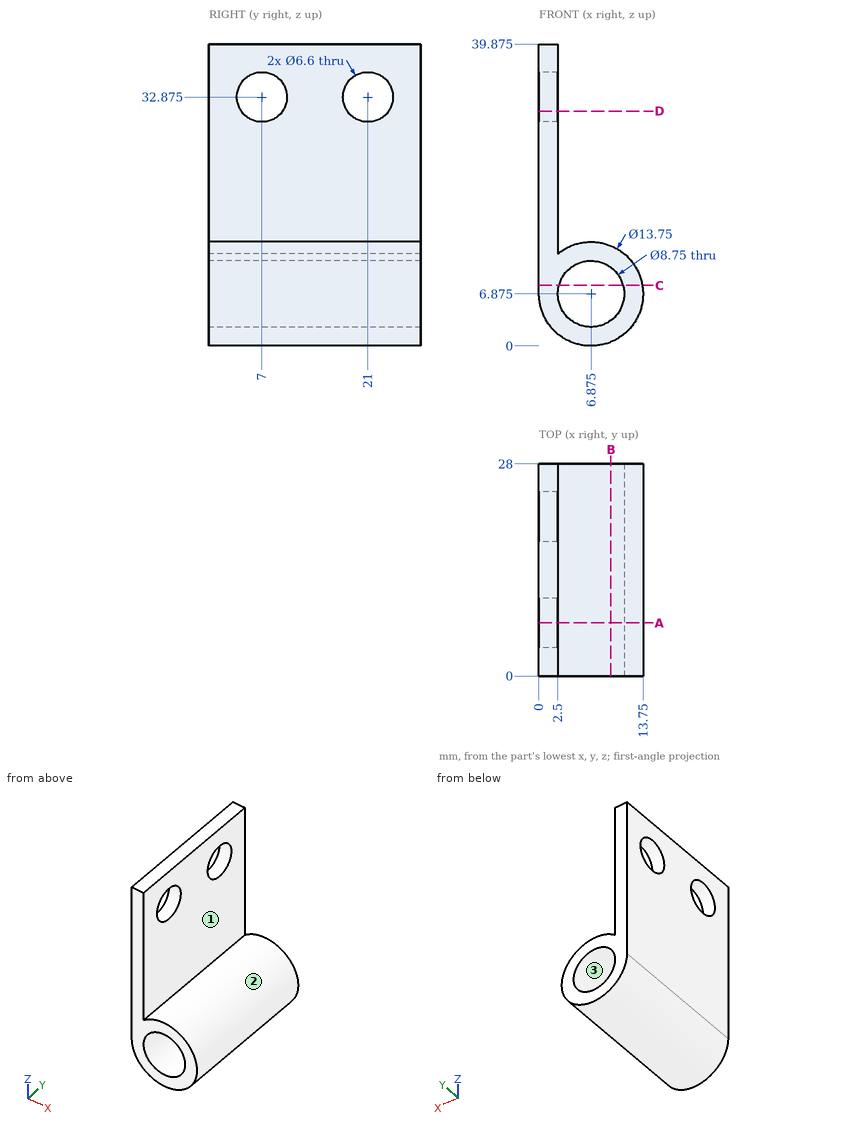
Geometry: see drawing. Coordinates: mm, zero at the bounding-box minimum. Give positions to 0.01 mm unless a question says otherwise; leave off trailing zeros. Write each loop counter-clockwise with the first axis right and the second up, starting at its lowest first coordinate (ties: lowest second). Pieces come first, ordered by that corner, then holes. Notation, with made-up numbers: M 35,33.25 L 57,33.25 A37 cw 57,72.25 Z; hole C -33,0 d5. An arc over 180 degrees is marked long. Answer in a Markdown table with one row per item. Add a question column.
(1) Mould query, pull axis Z, two halves, no side actions, for the marked faces 1, 2 and 3. Classes: +Z half, -Z half, draft (parallel to the pull), parting line (faces both ways), or undercut.
(2) Ray query, line 1 (X direction, y = 16, z = 34.5); line 2 (Z direction, x = 7, y = 23.5); line 3 (Z direction, x = 4, y = 19.5). Return the intervals inside material, ascending.
(3) Section B-B on x = 9.5. Return loops of the section in (y, z) (3 decimals).
(4) Section C-C on z = 8. Return loops of the section in (x, y), and give its area (3 significant figures).
(5) Section D-D on z = 31. Return loops of the section in (x, y), and give its area (3 significant figures).
(6) Section A-A on y = 7. Return loops of the section in (x, z) (3 decimals).
(7) First-contact query: pin 1 (7.5 mm diameter, centred on y = 21, z = 32.875, fed in from +X); pin 2 (1.5 mm diameter, centred on x = 10.5, y = 12, fed in from +Z); pin 3 (6 mm diameter, centred on y = 7, z = 32.875, fed in from +X) (3 decimals); pin 4 (1 mm diameter, centred on x = 5.5, y = 14, fed in from +Z). Flat tips, straight axial feed; report the tip coordinate or a pass-through.
Result set:
| question | item | result |
|---|---|---|
| 1 | face 1 | draft |
| 1 | face 2 | parting line |
| 1 | face 3 | undercut |
| 2 | line 1 | x = 0 to 2.5 |
| 2 | line 2 | z = 0 to 2.5, 11.25 to 13.75 |
| 2 | line 3 | z = 0.63 to 3.58, 10.17 to 13.12 |
| 3 | outline | M 0,0.521 L 28,0.521 L 28,3.375 L 0,3.375 Z; M 0,10.375 L 28,10.375 L 28,13.229 L 0,13.229 Z |
| 4 | outline | M 0,0 L 2.65,0 L 2.65,28 L 0,28 Z; M 11.1,0 L 13.66,0 L 13.66,28 L 11.1,28 Z |
| 4 | area | 146 mm^2 |
| 5 | outline | M 0,0 L 2.5,0 L 2.5,4.28 L 0,4.28 Z; M 0,9.72 L 2.5,9.72 L 2.5,18.28 L 0,18.28 Z; M 0,23.72 L 2.5,23.72 L 2.5,28 L 0,28 Z |
| 5 | area | 42.8 mm^2 |
| 6 | outline | M 0,6.875 A6.875 ccw long 2.5,12.178 L 2.5,29.575 L 0,29.575 Z; M 0,36.175 L 2.5,36.175 L 2.5,39.875 L 0,39.875 Z; hole C 6.875,6.875 d8.75 |
| 7 | pin 1 | stops at x = 2.5 |
| 7 | pin 2 | stops at z = 13.12 |
| 7 | pin 3 | passes through |
| 7 | pin 4 | stops at z = 13.69 |
